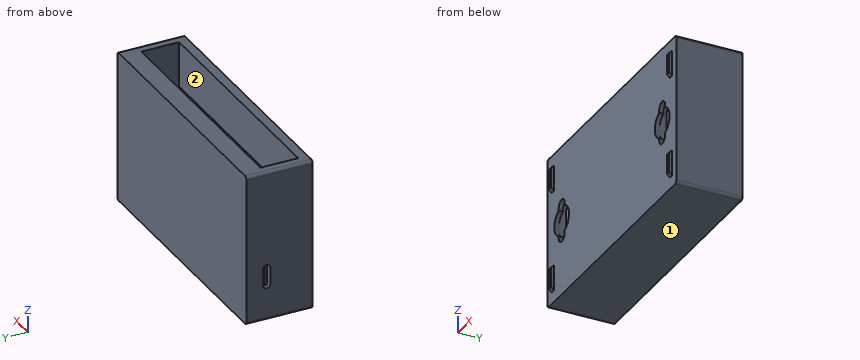
from build123d import *

# Parameters (mm, degrees)
SKETCH1_W                        = 88
SKETCH1_H                        = 52.7
BOSS_EXTRUDE1_DEPTH              = 23
SKETCH2_W                        = 81.25
SKETCH2_H                        = 13.1
CUT_EXTRUDE1_DEPTH               = 15.75
CUT_EXTRUDE2_DEPTH               = 6.5
SKETCH4_W                        = 6.69
SKETCH4_H                        = 0.8
BOSS_EXTRUDE2_DEPTH              = 6
FILLET1_R                        = 1
SKETCH6_W                        = 1.5
SKETCH6_H                        = 9
BOSS_EXTRUDE3_DEPTH              = 1
CHAMFER1_SIZE                    = 1
CHAMFER1_OF_SKETCH_PATTERN1_SIZE = 1
CUT_EXTRUDE3_DEPTH               = 4
CUT_EXTRUDE4_START               = -1.5
CUT_EXTRUDE4_DEPTH               = 2.5


with BuildPart() as part:
    # Sketch1 → Boss-Extrude1 (new body)
    with BuildSketch(Plane(origin=(0, 0, 0), x_dir=(1, 0, 0), z_dir=(0, 1, 0))):
        with Locations((44, 26.35)):
            Rectangle(SKETCH1_W, SKETCH1_H)
    extrude(amount=BOSS_EXTRUDE1_DEPTH)

    # Sketch2 → Cut-Extrude1 (cut)
    with BuildSketch(Plane.XY):
        with Locations((44, 9.85)):
            Rectangle(SKETCH2_W, SKETCH2_H)
    extrude(amount=-CUT_EXTRUDE1_DEPTH, mode=Mode.SUBTRACT)

    # Sketch3 → Cut-Extrude2 (cut)
    with BuildSketch(Plane.ZY):
        with BuildLine():
            ThreePointArc((-40.09, 17.28), (-41.37, 16), (-40.09, 14.72))
            Line((-40.09, 14.72), (-40.09, 17.28))
        make_face()
        with BuildLine():
            Line((-40.09, 17.28), (-40.09, 14.72))
            ThreePointArc((-40.09, 14.72), (-39.18490332, 15.09490332), (-38.81, 16))
            ThreePointArc((-38.81, 16), (-39.18490332, 16.90509668), (-40.09, 17.28))
        make_face()
        with BuildLine():
            ThreePointArc((-38.81, 16), (-39.18490332, 15.09490332), (-40.09, 14.72))
            Line((-40.09, 14.72), (-34.31, 14.72))
            ThreePointArc((-34.31, 14.72), (-35.59, 16), (-34.31, 17.28))
            Line((-34.31, 17.28), (-40.09, 17.28))
            ThreePointArc((-40.09, 17.28), (-39.18490332, 16.90509668), (-38.81, 16))
        make_face()
        with BuildLine():
            ThreePointArc((-34.31, 17.28), (-35.59, 16), (-34.31, 14.72))
            Line((-34.31, 14.72), (-34.31, 17.28))
        make_face()
        with BuildLine():
            Line((-34.31, 17.28), (-34.31, 14.72))
            ThreePointArc((-34.31, 14.72), (-33.40490332, 15.09490332), (-33.03, 16))
            ThreePointArc((-33.03, 16), (-33.40490332, 16.90509668), (-34.31, 17.28))
        make_face()
    extrude(amount=-CUT_EXTRUDE2_DEPTH, mode=Mode.SUBTRACT)

    # Sketch4 → Boss-Extrude2 (add)
    with BuildSketch(Plane.ZY.offset(-6.5)):
        with Locations((-37.2, 16)):
            Rectangle(SKETCH4_W, SKETCH4_H)
    extrude(amount=BOSS_EXTRUDE2_DEPTH)

    # Fillet1
    fillet1_edges = [part.edges().sort_by_distance(p)[0] for p in [
        (0, 11.5, -52.7),
        (88, 11.5, -52.7),
        (88, 11.5, 0),
        (0, 11.5, 0),
    ]]
    fillet(fillet1_edges, radius=FILLET1_R)

    # Sketch6 → Boss-Extrude3 (add)
    with BuildSketch(Plane.XZ):
        with Locations((3.75, -8.6)):
            Rectangle(SKETCH6_W, SKETCH6_H)
    boss_extrude3 = extrude(amount=BOSS_EXTRUDE3_DEPTH)

    # Chamfer1
    chamfer1_edges = [part.edges().sort_by_distance(p)[0] for p in [
        (3.75, -1, -4.1),
        (3.75, -1, -13.1),
    ]]
    chamfer(chamfer1_edges, length=CHAMFER1_SIZE - 0.0001)  # a hair under: the kernel refuses the full size

    # Sketch-Pattern1: Boss-Extrude3 at 3 more places
    with Locations((0, 0, -35.5), (80.5, 0, -35.5), (80.5, 0, 0)):
        add(boss_extrude3)

    # Chamfer1 of Sketch-Pattern1
    chamfer1_of_sketch_pattern1_edges = [part.edges().sort_by_distance(p)[0] for p in [
        (3.75, -1, -39.6),
        (3.75, -1, -48.6),
        (84.25, -1, -39.6),
        (84.25, -1, -48.6),
        (84.25, -1, -4.1),
        (84.25, -1, -13.1),
    ]]
    chamfer(chamfer1_of_sketch_pattern1_edges, length=CHAMFER1_OF_SKETCH_PATTERN1_SIZE - 0.0001)  # a hair under: the kernel refuses the full size

    # Sketch9 → Cut-Extrude3 (cut)
    with BuildSketch(Plane.XZ):
        with BuildLine():
            Line((11.75, -21.767424305), (11.75, -30.932575695))
            ThreePointArc((11.75, -30.932575695), (13.933300133, -29.088612788), (14.75, -26.35))
            ThreePointArc((14.75, -26.35), (13.933300133, -23.611387212), (11.75, -21.767424305))
        make_face()
        with BuildLine():
            Line((7.75, -21.767424305), (7.75, -30.932575695))
            ThreePointArc((7.75, -30.932575695), (9.75, -31.35), (11.75, -30.932575695))
            Line((11.75, -30.932575695), (11.75, -21.767424305))
            ThreePointArc((11.75, -21.767424305), (9.75, -21.35), (7.75, -21.767424305))
        make_face()
        with BuildLine():
            ThreePointArc((4.75, -26.35), (5.566699867, -29.088612788), (7.75, -30.932575695))
            Line((7.75, -30.932575695), (7.75, -21.767424305))
            ThreePointArc((7.75, -21.767424305), (5.566699867, -23.611387212), (4.75, -26.35))
        make_face()
        with BuildLine():
            Line((7.75, -20.85), (7.75, -21.767424305))
            ThreePointArc((7.75, -21.767424305), (9.75, -21.35), (11.75, -21.767424305))
            Line((11.75, -21.767424305), (11.75, -20.85))
            ThreePointArc((11.75, -20.85), (9.75, -18.85), (7.75, -20.85))
        make_face()
        with BuildLine():
            Line((7.75, -30.932575695), (7.75, -31.85))
            ThreePointArc((7.75, -31.85), (9.75, -33.85), (11.75, -31.85))
            Line((11.75, -31.85), (11.75, -30.932575695))
            ThreePointArc((11.75, -30.932575695), (9.75, -31.35), (7.75, -30.932575695))
        make_face()
    cut_extrude3 = extrude(amount=-CUT_EXTRUDE3_DEPTH, mode=Mode.SUBTRACT)

    # Sketch9<3> → Cut-Extrude4 (cut)
    with BuildSketch(Plane.XZ.offset(CUT_EXTRUDE4_START)):
        with BuildLine():
            ThreePointArc((11.75, -31.85), (9.75, -33.85), (7.75, -31.85))
            Line((7.75, -31.85), (7.75, -30.932575695))
            ThreePointArc((7.75, -30.932575695), (5.566699867, -29.088612788), (4.75, -26.35))
            Line((4.75, -26.35), (4.75, -31.85))
            ThreePointArc((4.75, -31.85), (9.75, -36.85), (14.75, -31.85))
            Line((14.75, -31.85), (14.75, -26.35))
            ThreePointArc((14.75, -26.35), (13.933300133, -29.088612788), (11.75, -30.932575695))
            Line((11.75, -30.932575695), (11.75, -31.85))
        make_face()
        with BuildLine():
            ThreePointArc((4.75, -26.35), (5.566699867, -23.611387212), (7.75, -21.767424305))
            Line((7.75, -21.767424305), (7.75, -20.85))
            ThreePointArc((7.75, -20.85), (9.75, -18.85), (11.75, -20.85))
            Line((11.75, -20.85), (11.75, -21.767424305))
            ThreePointArc((11.75, -21.767424305), (13.933300133, -23.611387212), (14.75, -26.35))
            Line((14.75, -26.35), (14.75, -20.85))
            ThreePointArc((14.75, -20.85), (9.75, -15.85), (4.75, -20.85))
            Line((4.75, -20.85), (4.75, -26.35))
        make_face()
    cut_extrude4 = extrude(amount=-CUT_EXTRUDE4_DEPTH, mode=Mode.SUBTRACT)

    # Sketch-Pattern2: Cut-Extrude3, Cut-Extrude4 at 1 more place
    with Locations((68.5, 0, 0)):
        add(cut_extrude3, mode=Mode.SUBTRACT)
        add(cut_extrude4, mode=Mode.SUBTRACT)


solid = part.part
Geometry: final body of the model. Coordinates: model frame, mm. Face numbers are marked on the shaded views. A direction names the side the tool comes from. Round coordinates to 2 decimals unless told otherwise and drop trailing zeros. Order: outer loops, then holes, each group sorted by start corner. A loop starts at its lowest first (then second) coordinate and runs counter-clockwise, first axis right, second up. Notation, with made-up numbers: (-34, 73) -> (-12, 73) arc R25 ccw to (-12, 87) -> close; hole circle Ø8 at (-11.5, 5.25). An arc over 180 degrees is marked (long way). Put each result on its own line as item: value. Start each with the question number.
Q1. Reachability of the marked faces 1 and 2 from +Z, -Z, +X, -X, +Y, -Y: full face, straight path, thin tool, end or side. Return the list, or none.
Q2. Section B-B on y = 8. Return the cut outline in (x, z) (3 decimals).
Q3. Line query: probe 1 along Y at (x, z) = (10, -16.5); probe 2 along X at (y, z) = (16.25, -5) (3 decimals); probe 3 along Y at (x, z) = (13, -8). Output: solid intervals per line, ascending.
Q4. Section D-D on x = 41.5. Return the cut outline in (y, z), and give its area (3 significant figures).
Q5. Section C-C on z = -29. Return the cut outline in (x, y), and give its area (3 significant figures).
Q6. Section A-A on x = 78.25. Return the cut outline in (y, z).
Q7. First-contact query: pin 1 (3 mm diameter, centred on x = 3, z = -37, fed in from -Y); pin 2 (1.3 mm diameter, centred on y = 15.5, z = -36, fed in from -X); pin 3 (0.5 mm diameter, centred on y = -0.5, z = -8.5, fed in from +X). Flat tips, straight axial feed; report the tip coordinate or a pass-through.
Ans:
1. face 1: -Z, +X, -X, +Y, -Y
1. face 2: +Z
2. outline: (0, -51.7) arc R1 ccw to (1, -52.7) -> (87, -52.7) arc R1 ccw to (88, -51.7) -> (88, -1) arc R1 ccw to (87, 0) -> (84.625, 0) -> (84.625, -15.75) -> (3.375, -15.75) -> (3.375, 0) -> (1, 0) arc R1 ccw to (0, -1) -> close
3. probe 1: y = 0 to 1.5, 4 to 23
3. probe 2: x = 0 to 3.375, 84.625 to 88
3. probe 3: y = 0 to 3.3, 16.4 to 23
4. outline: (0, -52.7) -> (23, -52.7) -> (23, 0) -> (16.4, 0) -> (16.4, -15.75) -> (3.3, -15.75) -> (3.3, 0) -> (0, 0) -> close
4. area: 1,010 mm2
5. outline: (0, 0) -> (5.51, 0) -> (5.51, 1.5) -> (4.75, 1.5) -> (4.75, 4) -> (14.75, 4) -> (14.75, 1.5) -> (13.99, 1.5) -> (13.99, 0) -> (74.01, 0) -> (74.01, 1.5) -> (73.25, 1.5) -> (73.25, 4) -> (83.25, 4) -> (83.25, 1.5) -> (82.49, 1.5) -> (82.49, 0) -> (88, 0) -> (88, 23) -> (0, 23) -> close
5. area: 1,950 mm2
6. outline: (0, -52.7) -> (23, -52.7) -> (23, 0) -> (16.4, 0) -> (16.4, -15.75) -> (3.3, -15.75) -> (3.3, 0) -> (0, 0) -> (0, -18.85) -> (1.5, -18.85) -> (1.5, -15.85) -> (4, -15.85) -> (4, -36.85) -> (1.5, -36.85) -> (1.5, -33.85) -> (0, -33.85) -> close
7. pin 1: stops at y = 0
7. pin 2: stops at x = 0.5
7. pin 3: stops at x = 85
